Part model, mm, in its own coordinate system. Face numbers are marked on the shaded views. A direction names the side the tool comes from. Give positions to 0.01 mm unless a question says otherwise; leave off trailing zeros. Order: outer loops, then holes, each group sorted by start corner. A loop starts at its lowest first (then second) coordinate and runs counter-clockwise, first axis right, second up. Notation, with made-up numbers: M 77,-8.75 L 124,-8.75 A29 ccw 124,20.25 Z; hole C 24.25,87.25 d4. An arc over 180 degrees is marked long. Answer as a JSON object with one key per item and string values.
from build123d import *

# Parameters (mm, degrees)
F0_R     = 1.5
F1_DEPTH = 1.5
F2_W     = 4.733152427
F2_H     = 7.5
F3_DEPTH = 3.7
F4_W     = 4.6442656718
F4_H     = 7.5
F5_DEPTH = 2.3
F6_R     = 0.2
F7_SIZE  = 0.2
F8_R     = 0.2


with BuildPart() as f1:
    # F0 (on Top) → F1 (new body)
    with BuildSketch(Plane.XY):
        Polygon((11.0012499681, 13.5), (-11.0012499681, 13.5), (-13.5, 11.0012499681), (-13.5, -11.0012499681), (-11.0012499681, -13.5), (11.0012499681, -13.5), (13.5, -11.0012499681), (13.5, 11.0012499681), align=None)
        with Locations((-10, -10)):
            Circle(F0_R, mode=Mode.SUBTRACT)
        with Locations((10, -10)):
            Circle(F0_R, mode=Mode.SUBTRACT)
        with Locations((-10, 10)):
            Circle(F0_R, mode=Mode.SUBTRACT)
        with Locations((10, 10)):
            Circle(F0_R, mode=Mode.SUBTRACT)
    extrude(amount=F1_DEPTH)

    # F2 (on face) → F3 (join)
    with BuildSketch(Plane.XY.offset(1.5)):
        with Locations((-11.6115645505, -2.75)):
            Rectangle(F2_W, F2_H)
    extrude(amount=F3_DEPTH)

    # F4 (on face) → F5 (join)
    with BuildSketch(Plane(origin=(0, 0, 0), x_dir=(1, 0, 0), z_dir=(0, 0, -1))):
        with Locations((-11.5750247117, 3.75)):
            Rectangle(F4_W, F4_H)
    extrude(amount=F5_DEPTH)

    # F6
    f6_edges = [f1.edges().sort_by_distance(p)[0] for p in [
        (-11.611565, 1, 5.2),
        (-9.244988, -2.75, 5.2),
        (-11.611565, -6.5, 5.2),
        (-9.244988, -6.5, 3.35),
        (-9.244988, 1, 3.35),
        (-13.978141, -2.75, 5.2),
        (-13.978141, -6.5, 3.35),
        (-13.978141, 1, 3.35),
    ]]
    fillet(f6_edges, radius=F6_R)

    # F7
    f7_edges = [f1.edges().sort_by_distance(p)[0] for p in [
        (0, -13.5, 1.5),
        (-12.250625, -12.250625, 1.5),
        (-13.5, -8.750625, 1.5),
        (12.250625, -12.250625, 1.5),
        (13.5, 0, 1.5),
        (-13.5, 6.000625, 1.5),
        (-12.250625, 12.250625, 1.5),
        (0, 13.5, 1.5),
        (12.250625, 12.250625, 1.5),
        (13.5, 0, 0),
        (0, 13.5, 0),
        (-12.250625, 12.250625, 0),
        (-13.5, 5.500625, 0),
        (-13.5, -9.250625, 0),
        (-12.250625, -12.250625, 0),
        (0, -13.5, 0),
        (12.250625, -12.250625, 0),
    ]]
    chamfer(f7_edges, length=F7_SIZE)

    # F8
    f8_edges = [f1.edges().sort_by_distance(p)[0] for p in [
        (-11.575025, -7.5, -2.3),
        (-9.252892, -3.75, -2.3),
        (-11.575025, 0, -2.3),
        (-13.897158, 0, -1.15),
        (-13.897158, -7.5, -1.15),
        (-9.252892, -7.5, -1.15),
        (-9.252892, 0, -1.15),
    ]]
    fillet(f8_edges, radius=F8_R)


solid = f1.part
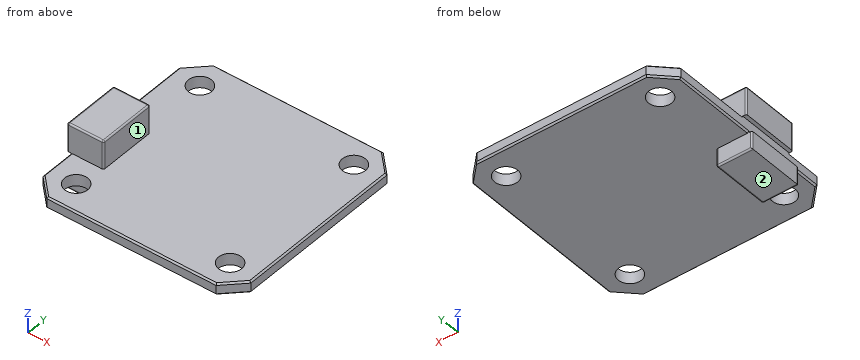
1. Cut at A-A on x = -10. Give the cut face in (y, z).
Worked answers:
{"outline": "M -13.5,0.2 L -13.3,0 L -11.5,0 L -11.5,1.5 L -13.3,1.5 L -13.5,1.3 Z; M -8.5,0 L -7.5,0 L -7.5,-2.1 A0.2 ccw -7.3,-2.3 L -0.2,-2.3 A0.2 ccw 0,-2.1 L 0,0 L 8.5,0 L 8.5,1.5 L 1,1.5 L 1,5 A0.2 ccw 0.8,5.2 L -6.3,5.2 A0.2 ccw -6.5,5 L -6.5,1.5 L -8.5,1.5 Z; M 11.5,0 L 13.3,0 L 13.5,0.2 L 13.5,1.3 L 13.3,1.5 L 11.5,1.5 Z"}
2. Which spindle directions (+Z, -Z, +X, -X, +Y, -Y) get a long thin tool onto all of the face, cutting with end or side? Do the marked faces 1 and 2. Say none if no direction does.
Worked answers:
{"face 1": "+Z, +X, +Y, -Y", "face 2": "-Z, +X, -X, +Y, -Y"}
3. Cut at D-D on x = 1.25. Give the cut face in (y, z), plus the area to 3 significant figures.
Worked answers:
{"outline": "M -13.5,0.2 L -13.3,0 L 13.3,0 L 13.5,0.2 L 13.5,1.3 L 13.3,1.5 L -13.3,1.5 L -13.5,1.3 Z", "area": "40.4 mm^2"}
4. Cut at B-B on y = 10. Give the cut face in (x, z).
Worked answers:
{"outline": "M -13.5,0.2 L -13.3,0 L -11.5,0 L -11.5,1.5 L -13.3,1.5 L -13.5,1.3 Z; M -8.5,0 L 8.5,0 L 8.5,1.5 L -8.5,1.5 Z; M 11.5,0 L 13.3,0 L 13.5,0.2 L 13.5,1.3 L 13.3,1.5 L 11.5,1.5 Z"}
5. Pin check, flat tips, straight feed: P1, Ø1.8, axis at x = -11, z = 4, coming from the +Y side; P2, Ø1.8, axis at x = -12.5, z = -1.5, coming from the -Y side; P3, Ø1.5, axis at y = 2, z = 2.5, coming from the -X side; P4, Ø1.8, axis at y = -2.5, z = -1, coming from the -X side. Stop position of each tip, or through.
Worked answers:
{"P1": "stops at y = 1", "P2": "stops at y = -7.5", "P3": "passes through", "P4": "stops at x = -13.9"}
6. Cut at C-C on z = 2.5. Give the cut face in (x, y).
Worked answers:
{"outline": "M -13.98,-6.3 A0.2 ccw -13.78,-6.5 L -9.44,-6.5 A0.2 ccw -9.24,-6.3 L -9.24,0.8 A0.2 ccw -9.44,1 L -13.78,1 A0.2 ccw -13.98,0.8 Z"}
7. Probe line 1 along Y through (x, z) = (10, 0.85); line 2 along Z through (x, y) = (1, 2.5); line 3 along Y through (x, z) = (-11.5, 2.5). List the from-to ranges inside material, lowest first.
Worked answers:
{"line 1": "y = -13.5 to -11.5, -8.5 to 8.5, 11.5 to 13.5", "line 2": "z = 0 to 1.5", "line 3": "y = -6.5 to 1"}
